For this review, take the finished solid that the model builds, in its own axes (mm). Round coordinates to 2 decimals unless told otherwise and drop trailing zeros. Loops run counter-clockwise (first coordinate to the right, second up) from the corner with the lowest first, then second, coordinate; pieces in that order, holes last. Notation, with made-up numbers: M -16,81.25 L 7,81.25 A34 cw 7,119.25 Z; hole C 34.25,-31.5 d11. An arc over 180 degrees is marked long. One line per question, with ' | ' between items. Start each with the question number.
1) For probe 1 along Z at (x, y) = (606, 1642.5); probe 2 along Z at (x, y) = (608.5, 1642.75); probe 3 along Z at (x, y) = (547.5, 1645.75), list the stretches that pass through material, from the lowest coordinate up. Write a range as from..to.
2) For pin 1 Ø2 at (y, z) = (1646.5, 1383) entering from -X; pin 2 Ø1.5 at (y, z) = (1648, 1466.5) entering from +X; pin 3 Ø4 at (x, y) = (575.5, 1647) entering from +Z; pin 4 Ø16 at (x, z) = (543.21, 1480.1) entering from -Y, all flat-tipped, find the tip position at first contact; note any pin that passes through.
3) We need section D-D (z = 1434). Give the boundary of the cut face in (x, y).
4) We need section B-B (y = 1645). Give the boundary of the cut face in (x, z).
5) We need section A-A (x = 602.5). Give the boundary of the cut face in (y, z).
6) We need section C-C (x = 547). Give the boundary of the cut face in (y, z), and give its area (3 significant figures).
```python
from build123d import *

# Parameters (mm, degrees)
SKETCH1_W           = 62.7
SKETCH1_H           = 113.5
BOSS_EXTRUDE1_DEPTH = 8
SKETCH2_R           = 7.5
BOSS_EXTRUDE2_DEPTH = 8
SKETCH3_R           = 5
CUT_EXTRUDE1_DEPTH  = 8


with BuildPart() as part:
    # Sketch1 → Boss-Extrude1 (new body)
    with BuildSketch(Plane(origin=(-3.563e-06, 1641.987881811, -1.519e-06), x_dir=(0.999999999, 2e-09, 3.7953e-05), z_dir=(-2e-09, 1, -1e-09))):
        with Locations((574.61782777, -1423.325985679)):
            Rectangle(SKETCH1_W, SKETCH1_H)
    extrude(amount=BOSS_EXTRUDE1_DEPTH)

    # Sketch2 → Boss-Extrude2 (add)
    with BuildSketch(Plane(origin=(-3.563e-06, 1641.987881811, -1.519e-06), x_dir=(0.999999999, 2e-09, 3.7953e-05), z_dir=(2e-09, -1, 1e-09))):
        with Locations((543.26782777, 1366.575985679)):
            Circle(SKETCH2_R)
        with Locations((605.96782777, 1366.575985679)):
            Circle(SKETCH2_R)
        with Locations((605.96782777, 1480.075985679)):
            Circle(SKETCH2_R)
        with Locations((543.26782777, 1480.075985679)):
            Circle(SKETCH2_R)
    extrude(amount=-BOSS_EXTRUDE2_DEPTH)

    # Sketch3 → Cut-Extrude1 (cut)
    with BuildSketch(Plane(origin=(-3.563e-06, 1641.987881811, -1.519e-06), x_dir=(0.999999999, 2e-09, 3.7953e-05), z_dir=(2e-09, -1, 1e-09))):
        with Locations((543.26782777, 1480.075985679)):
            Circle(SKETCH3_R)
        with Locations((605.96782777, 1480.075985679)):
            Circle(SKETCH3_R)
        with Locations((605.96782777, 1366.575985679)):
            Circle(SKETCH3_R)
        with Locations((543.26782777, 1366.575985679)):
            Circle(SKETCH3_R)
    extrude(amount=-CUT_EXTRUDE1_DEPTH, mode=Mode.SUBTRACT)


solid = part.part
```
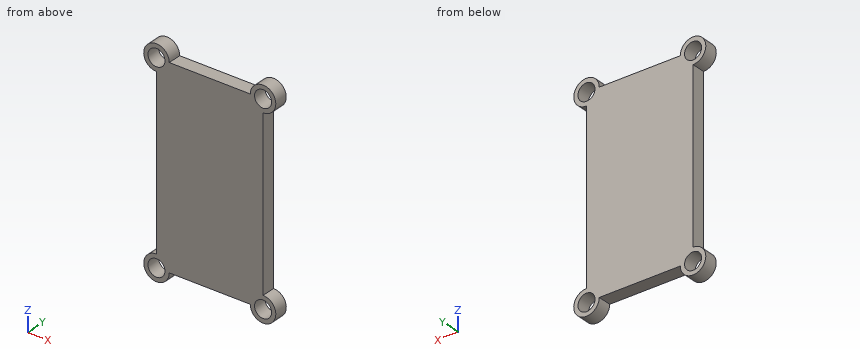
Answers below:
1) probe 1: 1359.1..1361.6, 1371.6..1374.1, 1472.6..1475.1, 1485.1..1487.6 | probe 2: 1359.56..1362.32, 1370.88..1373.64, 1473.06..1475.82, 1484.38..1487.14 | probe 3: 1360.44..1364.02, 1369.17..1477.53, 1482.67..1486.25
2) pin 1: x = 543.22 | pin 2: x = 605.91 | pin 3: z = 1480.1 | pin 4: y = 1641.99
3) outline: M 543.21,1641.99 L 605.91,1641.99 L 605.91,1649.99 L 543.21,1649.99 Z
4) outline: M 543.21,1472.6 L 543.22,1374.1 A7.5 ccw long 550.72,1366.6 L 598.42,1366.6 A7.5 ccw long 605.92,1374.1 L 605.91,1472.6 A7.5 ccw long 598.41,1480.1 L 550.71,1480.1 A7.5 ccw long Z; hole C 543.21,1480.1 d10; hole C 543.22,1366.6 d10; hole C 605.91,1480.1 d10; hole C 605.92,1366.6 d10
5) outline: M 1641.99,1359.92 L 1649.99,1359.92 L 1649.99,1362.95 L 1641.99,1362.95 Z; M 1641.99,1370.25 L 1649.99,1370.25 L 1649.99,1476.44 L 1641.99,1476.44 Z; M 1641.99,1483.75 L 1649.99,1483.75 L 1649.99,1486.78 L 1641.99,1486.78 Z
6) outline: M 1641.99,1360.12 L 1649.99,1360.12 L 1649.99,1363.33 L 1641.99,1363.33 Z; M 1641.99,1369.86 L 1649.99,1369.86 L 1649.99,1476.83 L 1641.99,1476.83 Z; M 1641.99,1483.36 L 1649.99,1483.36 L 1649.99,1486.57 L 1641.99,1486.57 Z | area: 907 mm^2
